Build history of the part. All positions in model axes, mm. Give positions to 0.01 mm unless a question says otherwise; leave off trailing zeros. Loops run counter-clockwise (first coordinate to the right, second up) from the corner with the lowest first, then second, coordinate; pieces in that order, holes last. Notation, with made-up numbers: M 28.25,33 L 66.25,33 A22 cw 66.25,44 Z; hole C 31,42 d4. An arc over 180 degrees is marked long. Answer as a JSON object with one key per item and string values. Group by question number.
1. Drop flat-ended pins along their axis: pin 1 Ø12 at (x, z) = (-3, 3) entering from -Y; pin 2 Ø4 at (x, z) = (-6, -9) entering from +Y. Give the stop position or say it passes through.
2. Drill centre lines: line 1 along Y through (x, z) = (0.5, -7.75); line 2 along X through (y, z) = (226, 10); line 3 along Y through (x, z) = (2.5, 2.5). Where is each one in solid material? Low to high. Write a range as [from, to].
3. Slice it at B-B (x = 7.25). List the corners of the cut face in (y, z), then the cut area to 3 significant figures.
4. Slice it at A-A (z = -6.25). List the corners of the cut face in (x, y), then the cut area to 3 significant figures.
from build123d import *

# Parameters (mm, degrees)
ESQUISSE1_W        = 25
ESQUISSE1_H        = 25
BOSS_EXTRU_1_DEPTH = 225
BOSS_EXTRU_2_DEPTH = 25
BOSS_EXTRU_3_DEPTH = 25


with BuildPart() as part:
    # Esquisse1 → Boss.-Extru.1 (new body)
    with BuildSketch(Plane(origin=(0, 0, 0), x_dir=(1, 0, 0), z_dir=(0, 1, 0))):
        Rectangle(ESQUISSE1_W, ESQUISSE1_H)
    extrude(amount=BOSS_EXTRU_1_DEPTH)

    # Esquisse2 → Boss.-Extru.2 (add)
    with BuildSketch(Plane.XY.offset(12.5)):
        with BuildLine():
            Line((-12.5, 225), (12.5, 225))
            ThreePointArc((12.5, 225), (0, 237.5), (-12.5, 225))
        make_face()
    extrude(amount=-BOSS_EXTRU_2_DEPTH)

    # Esquisse3 → Boss.-Extru.3 (add)
    with BuildSketch(Plane.XY.offset(12.5)):
        with BuildLine():
            Line((-12.5, 0), (12.5, 0))
            ThreePointArc((12.5, 0), (0, -12.5), (-12.5, 0))
        make_face()
    extrude(amount=-BOSS_EXTRU_3_DEPTH)


solid = part.part
Established:
{
 "1": {"pin 1": "stops at y = -12.5", "pin 2": "stops at y = 236.84"},
 "2": {"line 1": "y = [-12.49, 237.49]", "line 2": "x = [-12.46, 12.46]", "line 3": "y = [-12.25, 237.25]"},
 "3": {"outline": "M -10.18,-12.5 L 235.18,-12.5 L 235.18,12.5 L -10.18,12.5 Z", "area": "6,130 mm^2"},
 "4": {"outline": "M -12.5,0 A12.5 ccw 12.5,0 L 12.5,225 A12.5 ccw -12.5,225 Z", "area": "6,120 mm^2"}
}
